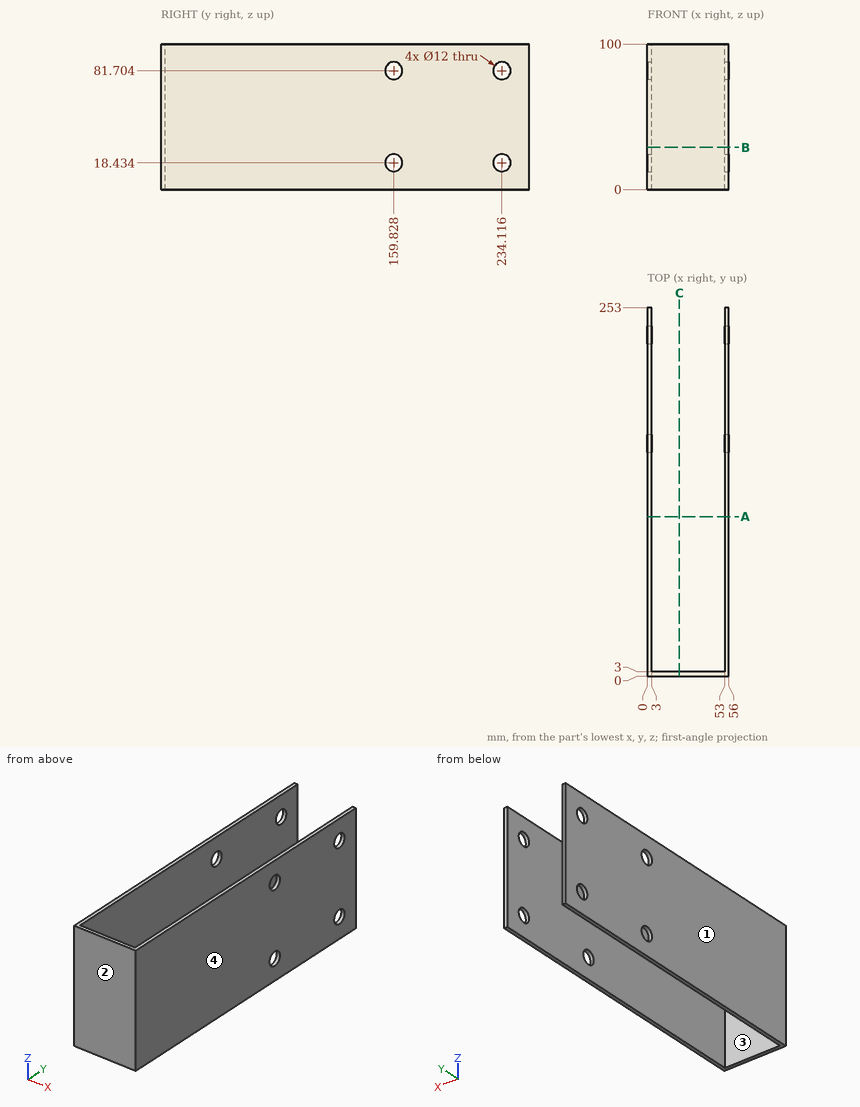
Geometry: see drawing. Coordinates: mm, zero at the bounding-box minimum. Round coordinates to 2 decimals unless told otherwise and drop trailing zeros. Order: outer loops, then holes, each group sorted by start corner. A loop starts at its lowest first (then second) coordinate and runs counter-clockwise, first axis right, second up. Notation, with made-up numbers: (56, 42.25) -> (65, 42.25) arc R27 ccw to (65, 79.25) -> close; hole circle Ø8 at (70.25, -29). An arc over 180 degrees is marked (long way). Use CSV: the item, a comma, the result in double quotes.
(1) Section C-C on x = 22. Return the cut outline in (y, z).
Report:
outline,"(0, 0) -> (3, 0) -> (3, 100) -> (0, 100) -> close"
(2) First-contact query: pin 1 Ø12 at (x, z) = (30.5, 51) entering from +Y. Flat tip, straight axial feed; report the tip coordinate or a pass-through.
Report:
pin 1,"y = 3"
(3) Section A-A on y = 109.5. Return the cut outline in (x, z), and give its area (3 significant figures).
Report:
outline,"(0, 0) -> (3, 0) -> (3, 100) -> (0, 100) -> close; (53, 0) -> (56, 0) -> (56, 100) -> (53, 100) -> close"
area,"600 mm^2"
(4) Section B-B on z = 29. Return the cut outline in (x, y).
Report:
outline,"(0, 0) -> (56, 0) -> (56, 253) -> (53, 253) -> (53, 3) -> (3, 3) -> (3, 253) -> (0, 253) -> close"
(5) Pull-direction query (X, two-part tool) for the marked faces 1, 2, 3 and 4; classes: +X half, -X half, draft (parallel to the pull), parting line (faces both ways), or undercut.
Report:
face 1,"-X half"
face 2,"draft"
face 3,"undercut"
face 4,"+X half"
(6) Ray query, L1, parallel to X at y = 136.5, z = 18; L2, parallel to Y at x = 12.5, z = 90.5. Return the intervals inside material, ascending.
Report:
L1,"0 to 3, 53 to 56"
L2,"0 to 3"
